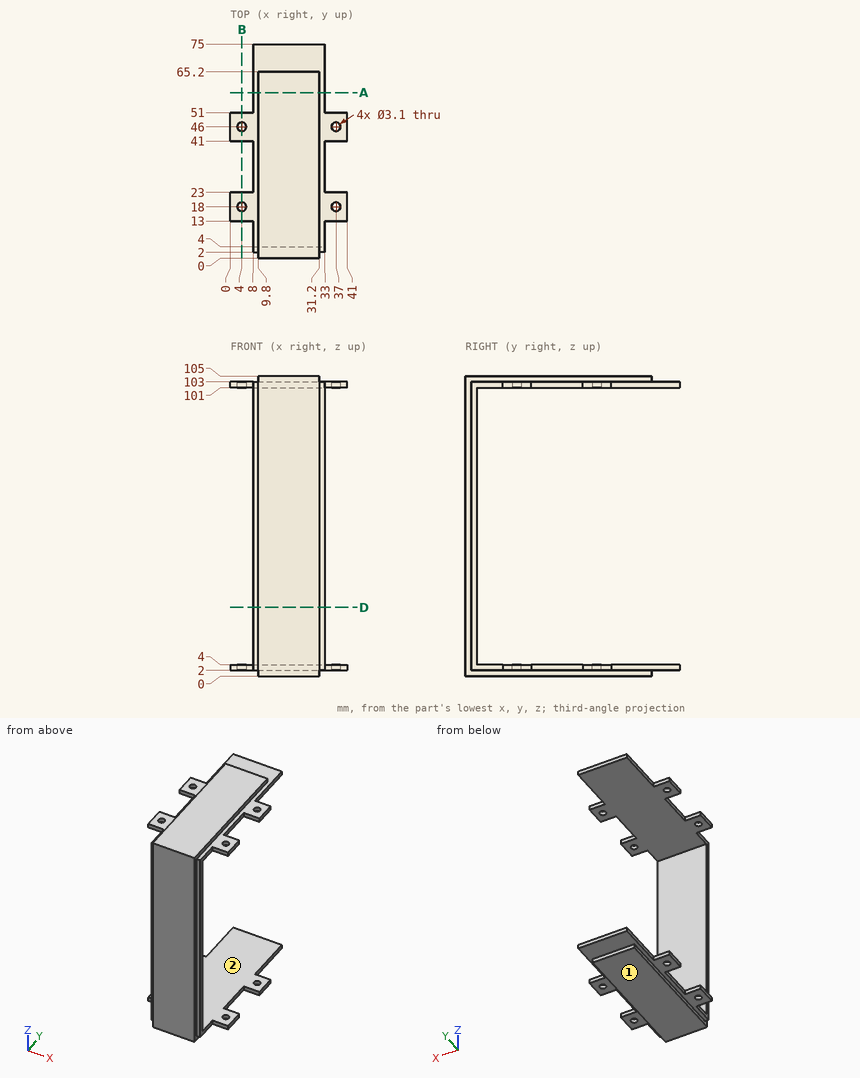
Source: three-view drawing plus pictorial views. Frame: mm from the lowest corner of the part. A direction names the side the tool comes from. Coordinates: 2 decimals unless noted, no trailing zeros. Loops run counter-clockwise (first coordinate to the right, second up) from the corner with the lowest first, then second, coordinate; pieces in that order, holes last. Notation, with made-up numbers: (-38, 51.25) -> (-2, 51.25) arc R19 cw to (-2, 73.25) -> close; hole circle Ø10 at (86, 0.5). An arc over 180 degrees is marked (long way). One line per item, written item: value.
(1) Set-up query: the marked faces 1 and 2. Return all of +Z, -Z, +X, -X, +Y, -Y with unobstructed straight access to the full face (end or side cutting, diameter ignored); none if empty.
Answer below:
face 1: -Z, +X, -X, +Y, -Y
face 2: +X, -X, +Y
(2) Cut plane D-D (z = 24). Output: boundary loops of the cut face in (x, y), then the cut area to 3 significant figures.
Answer below:
outline: (8, 2) -> (9.8, 2) -> (9.8, 0) -> (31.2, 0) -> (31.2, 2) -> (33, 2) -> (33, 4) -> (8, 4) -> close
area: 92.8 mm2
(3) Ray query, line 1 along Y through (x, z) = (37, 3.55); line 2 along Z through (x, y) = (12.5, 45); line 3 along Z through (x, y) = (35, 48.5). Return the intervals inside material, ascending.
Answer below:
line 1: y = 13 to 16.45, 19.55 to 23, 41 to 44.45, 47.55 to 51
line 2: z = 0 to 4, 101 to 105
line 3: z = 2 to 4, 101 to 103
(4) Cut plane A-A (y = 58). Output: boundary loops of the cut face in (x, z).
Answer below:
outline: (8, 2) -> (9.8, 2) -> (9.8, 0) -> (31.2, 0) -> (31.2, 2) -> (33, 2) -> (33, 4) -> (8, 4) -> close; (8, 101) -> (33, 101) -> (33, 103) -> (31.2, 103) -> (31.2, 105) -> (9.8, 105) -> (9.8, 103) -> (8, 103) -> close
(5) Pin query (flat end, axial travel): pin 1 Ø2 at (x, z) = (37, 3) entering from -Y; pin 2 Ø0.6 at (x, z) = (5, 102.5) entering from +Y; pin 3 Ø4 at (x, z) = (24.5, 18.5) entering from +Y; pin 4 Ø3 at (x, y) = (37, 18) entering from +Z. Return the tip coordinate at first contact, or that it passes through.
Answer below:
pin 1: stops at y = 13
pin 2: stops at y = 51
pin 3: stops at y = 4
pin 4: passes through
(6) Cut plane B-B (x = 4). Give the number of separate pieces and of enclosed holes in the cut face, then the cut area to 3 significant figures.
Answer below:
separate pieces: 8
enclosed holes: 0
area: 55.2 mm2
